from build123d import *

# Parameters (mm, degrees)
F1_DEPTH = 100
F2_DEPTH = 1
F3_START = 99
F3_DEPTH = 1


with BuildPart() as f1:
    # F0 (on Top) → F1 (new body)
    with BuildSketch(Plane.XY):
        Polygon((-10.3999599814, 2), (-12.5, 2), (-12.5, -1.2), (-9.5, -1.2), (-9.5, 1.1444095289), (-9.5, 2), align=None)
        Polygon((-12.5, -1.2), (-12.5, 2), (-12.8442417498, 4), (-13.5327252493, 4), (-12.5, -2), align=None)
        Polygon((-12.8442417498, 4), (-12.5, 2), (-10.3999599814, 2), (-9.5, 2), (-9.8442417498, 4), align=None)
        Polygon((-13.5327252493, 4), (-12.8442417498, 4), (-13.1884834996, 6), (-13.8769669991, 6), align=None)
        Polygon((-13.5327252493, 8), (-13.1884834996, 6), (-10.1884834996, 6), (-10.5327252493, 8), align=None)
        Polygon((-13.8769669991, 6), (-13.1884834996, 6), (-13.5327252493, 8), (-14.2212087489, 8), align=None)
        Polygon((-14.2212087489, 8), (-13.5327252493, 8), (-13.8769669991, 10), (-14.5654504987, 10), align=None)
        Polygon((-14.2212087489, 12), (-13.8769669991, 10), (-10.8769669991, 10), (-11.2212087489, 12), align=None)
        Polygon((-14.9096922485, 16), (-14.5654504987, 14), (-11.5654504987, 14), (-11.9096922485, 16), align=None)
        Polygon((-15.598175748, 20), (-15.2539339983, 18), (-12.2539339983, 18), (-12.598175748, 20), align=None)
        Polygon((-14.5654504987, 10), (-13.8769669991, 10), (-14.2212087489, 12), (-14.9096922485, 12), align=None)
        Polygon((-14.9096922485, 12), (-14.2212087489, 12), (-14.5654504987, 14), (-15.2539339983, 14), align=None)
        Polygon((-15.2539339983, 14), (-14.5654504987, 14), (-14.9096922485, 16), (-15.598175748, 16), align=None)
        Polygon((-15.598175748, 16), (-14.9096922485, 16), (-15.2539339983, 18), (-15.9424174978, 18), align=None)
        Polygon((-15.9424174978, 18), (-15.2539339983, 18), (-15.598175748, 20), (-16.2866592476, 20), align=None)
        Polygon((-16.2866592476, 20), (-15.598175748, 20), (-15.9424174978, 22), (-16.6309009974, 22), align=None)
        Polygon((-16.6309009974, 22), (-15.9424174978, 22), (-16.2866592476, 24), (-16.9751427472, 24), align=None)
        Polygon((-16.9751427472, 24), (-16.2866592476, 24), (-16.6309009974, 26), (-17.319384497, 26), align=None)
        Polygon((-17.319384497, 26), (-16.6309009974, 26), (-13.6309009974, 26), (-13.6309009974, 27.8660617122), (-17.319384497, 27.8660617122), align=None)
        Polygon((-16.2866592476, 24), (-15.9424174978, 22), (-12.9424174978, 22), (-13.2866592476, 24), align=None)
    extrude(amount=F1_DEPTH)

    # F0 (on Top) → F2 (join)
    with BuildSketch(Plane.XY):
        Polygon((-12.8442417498, 4), (-12.5, 2), (-10.3999599814, 2), (-9.5, 2), (-9.8442417498, 4), align=None)
        Polygon((-12.5, -1.2), (-12.5, 2), (-12.8442417498, 4), (-13.5327252493, 4), (-12.5, -2), align=None)
        Polygon((-13.1884834996, 6), (-12.8442417498, 4), (-9.8442417498, 4), (-10.1884834996, 6), align=None)
        Polygon((-13.5327252493, 4), (-12.8442417498, 4), (-13.1884834996, 6), (-13.8769669991, 6), align=None)
        Polygon((-13.5327252493, 8), (-13.1884834996, 6), (-10.1884834996, 6), (-10.5327252493, 8), align=None)
        Polygon((-13.8769669991, 6), (-13.1884834996, 6), (-13.5327252493, 8), (-14.2212087489, 8), align=None)
        Polygon((-13.8769669991, 10), (-13.5327252493, 8), (-10.5327252493, 8), (-10.8769669991, 10), align=None)
        Polygon((-14.2212087489, 8), (-13.5327252493, 8), (-13.8769669991, 10), (-14.5654504987, 10), align=None)
        Polygon((-14.2212087489, 12), (-13.8769669991, 10), (-10.8769669991, 10), (-11.2212087489, 12), align=None)
        Polygon((-14.5654504987, 10), (-13.8769669991, 10), (-14.2212087489, 12), (-14.9096922485, 12), align=None)
        Polygon((-14.5654504987, 14), (-14.2212087489, 12), (-11.2212087489, 12), (-11.5654504987, 14), align=None)
        Polygon((-14.9096922485, 12), (-14.2212087489, 12), (-14.5654504987, 14), (-15.2539339983, 14), align=None)
        Polygon((-14.9096922485, 16), (-14.5654504987, 14), (-11.5654504987, 14), (-11.9096922485, 16), align=None)
        Polygon((-15.2539339983, 14), (-14.5654504987, 14), (-14.9096922485, 16), (-15.598175748, 16), align=None)
        Polygon((-15.2539339983, 18), (-14.9096922485, 16), (-11.9096922485, 16), (-12.2539339983, 18), align=None)
        Polygon((-15.598175748, 16), (-14.9096922485, 16), (-15.2539339983, 18), (-15.9424174978, 18), align=None)
        Polygon((-15.598175748, 20), (-15.2539339983, 18), (-12.2539339983, 18), (-12.598175748, 20), align=None)
        Polygon((-15.9424174978, 18), (-15.2539339983, 18), (-15.598175748, 20), (-16.2866592476, 20), align=None)
        Polygon((-15.9424174978, 22), (-15.598175748, 20), (-12.598175748, 20), (-12.9424174978, 22), align=None)
        Polygon((-16.2866592476, 20), (-15.598175748, 20), (-15.9424174978, 22), (-16.6309009974, 22), align=None)
        Polygon((-16.2866592476, 24), (-15.9424174978, 22), (-12.9424174978, 22), (-13.2866592476, 24), align=None)
        Polygon((-16.6309009974, 22), (-15.9424174978, 22), (-16.2866592476, 24), (-16.9751427472, 24), align=None)
        Polygon((-16.6309009974, 26), (-16.2866592476, 24), (-13.2866592476, 24), (-13.6309009974, 26), align=None)
        Polygon((-16.9751427472, 24), (-16.2866592476, 24), (-16.6309009974, 26), (-17.319384497, 26), align=None)
        Polygon((-17.319384497, 26), (-16.6309009974, 26), (-13.6309009974, 26), (-13.6309009974, 27.8660617122), (-17.319384497, 27.8660617122), align=None)
    extrude(amount=F2_DEPTH)

    # F0 (on Top) → F3 (join)
    with BuildSketch(Plane.XY.offset(F3_START)):
        Polygon((-12.8442417498, 4), (-12.5, 2), (-10.3999599814, 2), (-9.5, 2), (-9.8442417498, 4), align=None)
        Polygon((-10.3999599814, 2), (-12.5, 2), (-12.5, -1.2), (-9.5, -1.2), (-9.5, 1.1444095289), (-9.5, 2), align=None)
        Polygon((-12.5, -1.2), (-12.5, 2), (-12.8442417498, 4), (-13.5327252493, 4), (-12.5, -2), align=None)
        Polygon((-13.1884834996, 6), (-12.8442417498, 4), (-9.8442417498, 4), (-10.1884834996, 6), align=None)
        Polygon((-13.5327252493, 4), (-12.8442417498, 4), (-13.1884834996, 6), (-13.8769669991, 6), align=None)
        Polygon((-13.5327252493, 8), (-13.1884834996, 6), (-10.1884834996, 6), (-10.5327252493, 8), align=None)
        Polygon((-13.8769669991, 6), (-13.1884834996, 6), (-13.5327252493, 8), (-14.2212087489, 8), align=None)
        Polygon((-13.8769669991, 10), (-13.5327252493, 8), (-10.5327252493, 8), (-10.8769669991, 10), align=None)
        Polygon((-14.2212087489, 8), (-13.5327252493, 8), (-13.8769669991, 10), (-14.5654504987, 10), align=None)
        Polygon((-14.2212087489, 12), (-13.8769669991, 10), (-10.8769669991, 10), (-11.2212087489, 12), align=None)
        Polygon((-14.5654504987, 10), (-13.8769669991, 10), (-14.2212087489, 12), (-14.9096922485, 12), align=None)
        Polygon((-14.5654504987, 14), (-14.2212087489, 12), (-11.2212087489, 12), (-11.5654504987, 14), align=None)
        Polygon((-14.9096922485, 12), (-14.2212087489, 12), (-14.5654504987, 14), (-15.2539339983, 14), align=None)
        Polygon((-14.9096922485, 16), (-14.5654504987, 14), (-11.5654504987, 14), (-11.9096922485, 16), align=None)
        Polygon((-15.2539339983, 14), (-14.5654504987, 14), (-14.9096922485, 16), (-15.598175748, 16), align=None)
        Polygon((-15.2539339983, 18), (-14.9096922485, 16), (-11.9096922485, 16), (-12.2539339983, 18), align=None)
        Polygon((-15.598175748, 16), (-14.9096922485, 16), (-15.2539339983, 18), (-15.9424174978, 18), align=None)
        Polygon((-15.598175748, 20), (-15.2539339983, 18), (-12.2539339983, 18), (-12.598175748, 20), align=None)
        Polygon((-15.9424174978, 18), (-15.2539339983, 18), (-15.598175748, 20), (-16.2866592476, 20), align=None)
        Polygon((-15.9424174978, 22), (-15.598175748, 20), (-12.598175748, 20), (-12.9424174978, 22), align=None)
        Polygon((-16.2866592476, 20), (-15.598175748, 20), (-15.9424174978, 22), (-16.6309009974, 22), align=None)
        Polygon((-16.2866592476, 24), (-15.9424174978, 22), (-12.9424174978, 22), (-13.2866592476, 24), align=None)
        Polygon((-16.6309009974, 22), (-15.9424174978, 22), (-16.2866592476, 24), (-16.9751427472, 24), align=None)
        Polygon((-16.6309009974, 26), (-16.2866592476, 24), (-13.2866592476, 24), (-13.6309009974, 26), align=None)
        Polygon((-16.9751427472, 24), (-16.2866592476, 24), (-16.6309009974, 26), (-17.319384497, 26), align=None)
        Polygon((-17.319384497, 26), (-16.6309009974, 26), (-13.6309009974, 26), (-13.6309009974, 27.8660617122), (-17.319384497, 27.8660617122), align=None)
    extrude(amount=F3_DEPTH)


solid = f1.part
Here's how the part is built. I have some questions about the finished solid (model axes, mm). A direction names the side the tool comes from. Coordinates: 2 decimals unless noted, no trailing zeros. Answer in a Markdown table with one row per item.
(1) Thinking about a two-plate mould opening in Y: for faces 5 (the face through (-15, 27.866, 49)), 6 (the face through (-14, 21, 1)), 7 (the face through (-17.319, 27, 49)), which applies, +Y half, -Y half, draft (parallel to the pull), parting line (faces both ways), or undercut?
Answer key:
| item | result |
|---|---|
| face 5 | +Y half |
| face 6 | undercut |
| face 7 | draft |
(2) Will these pins go through, and if not, where does the flat tip stop? pin 1 Ø10 at (y, z) = (8.5, 83) entering from -X; pin 2 Ø5 at (y, z) = (12, 85) entering from -X; pin 3 Ø3 at (y, z) = (16.5, 14) entering from +X.
Answer key:
| item | result |
|---|---|
| pin 1 | x = -15.17 |
| pin 2 | x = -15.34 |
| pin 3 | x = -11.74 |
(3) On a 3-axis mill with a long thin cutter (end or side, diameter ignored), from which of +Z, -Z, +X, -X, +Y, -Y can I reach the whole of each face in a straight line? I mean faces 1 (the face through (-13.631, 27, 49)), 2 (the face through (-13, 13, 100)), 3 (the face through (-11, -1.2, 49)), 4 (the face through (-14, 18, 49)). Say none if no direction works.
Answer key:
| item | result |
|---|---|
| face 1 | +Z, -Z, +X, +Y |
| face 2 | +Z, +X, -X, +Y, -Y |
| face 3 | +Z, -Z, +X, -Y |
| face 4 | +X |
(4) Please list where these lines run through material, in increasing order: probe 1 along Z at (x, y) = (-11, 5.75); probe 2 along X at (y, z) = (8.5, 37); probe 3 along X at (y, z) = (0, 33.5).
Answer key:
| item | result |
|---|---|
| probe 1 | 0 to 1, 99 to 100 |
| probe 2 | -14.31 to -13.62 |
| probe 3 | -12.84 to -9.5 |
